Work out the finished part from the listing and answer in its coordinate system (mm). Face numbers are marked on the shaded views. A direction names the side the tool comes from. Coordinates: 2 decimals unless noted, no trailing zeros. Write each loop counter-clockwise with the first axis right and the second up, starting at its lowest first coordinate (ties: lowest second). Pieces come first, ordered by that corner, then holes. Notation, with made-up numbers: (56, 18) - (92, 18) arc R14 ccw to (92, 44) - close; hole circle Ø6 at (35.25, 58). An arc over 180 degrees is marked (long way). One line per item, written item: value.
```python
from build123d import *

# Parameters (mm, degrees)
F0_W     = 31.8
F0_H     = 15.8
F1_DEPTH = 9.6
F2_R     = 2.4
F3_DEPTH = 1.8
F4_T     = -1
F5_R     = 3.255
F5_R_2   = 2.4
F6_DEPTH = 8.6


# Not quite as in the source:
# - a pattern or mirror of a feature is missing from the dataset's text; its kind, count and spacing are read off the source's solid


with BuildPart() as f1:
    # F0 (on Top) → F1 (new body)
    with BuildSketch(Plane.XY):
        Rectangle(F0_W, F0_H)
    extrude(amount=F1_DEPTH)

    # F2 (on face) → F3 (join)
    with BuildSketch(Plane.XY.offset(9.6)):
        with Locations((-12, 4)):
            Circle(F2_R)
        with Locations((-4, 4)):
            Circle(F2_R)
        with Locations((4, 4)):
            Circle(F2_R)
        with Locations((12, 4)):
            Circle(F2_R)
    f3 = extrude(amount=F3_DEPTH)

    # F3_copies: F3 across plane
    add(f3.mirror(Plane(origin=(0, 0, 0), x_dir=(0, 0, -1), z_dir=(0, -1, 0))))

    # F4
    f4_openings = [f1.faces().sort_by_distance(p)[0] for p in [
        (0, 0, 0),
    ]]
    offset(amount=F4_T, openings=f4_openings, kind=Kind.INTERSECTION)

    # F5 (on face) → F6 (join, through all)
    with BuildSketch(Plane(origin=(0, 0, 8.6), x_dir=(1, 0, 0), z_dir=(0, 0, -1))):
        with Locations((-8, 0)):
            Circle(F5_R)
        with Locations((-8, 0)):
            Circle(F5_R_2, mode=Mode.SUBTRACT)
        Circle(F5_R)
        Circle(F5_R_2, mode=Mode.SUBTRACT)
        with Locations((8, 0)):
            Circle(F5_R)
        with Locations((8, 0)):
            Circle(F5_R_2, mode=Mode.SUBTRACT)
    extrude(amount=F6_DEPTH)


solid = f1.part
```
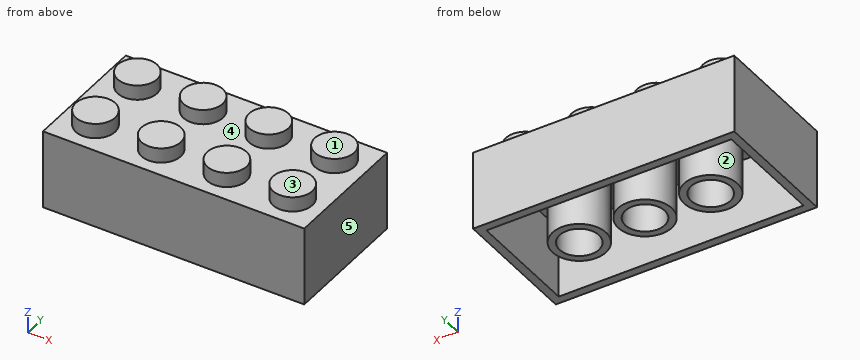
Item 1: Consider probe 1 along X at (y, z) = (4, 9.3); probe 2 along Y at (x, z) = (-8, 2.5) (3 decimals); probe 3 along Y at (x, z) = (12, 9.65). Determine where each line is inside the solid, lowest interval first.
Evaluation:
probe 1: x = -15.9 to -13.4, -10.6 to -5.4, -2.6 to 2.6, 5.4 to 10.6, 13.4 to 15.9
probe 2: y = -7.9 to -6.9, -3.255 to -2.4, 2.4 to 3.255, 6.9 to 7.9
probe 3: y = -6.4 to -5.4, -2.6 to -1.6, 1.6 to 2.6, 5.4 to 6.4
Item 2: Section A-A, the plane z = 6.5 is taken. Determine the outline of the cut face in (x, y) (3 decimals), then the cut area to 3 significant figures.
Evaluation:
outline: (-15.9, -7.9) - (15.9, -7.9) - (15.9, 7.9) - (-15.9, 7.9) - close; circle Ø6.51 at (-8, 0); circle Ø6.51 at (0, 0); circle Ø6.51 at (8, 0); hole (-14.9, -6.9) - (14.9, -6.9) - (14.9, 6.9) - (-14.9, 6.9) - close; hole circle Ø4.8 at (-8, 0); hole circle Ø4.8 at (0, 0); hole circle Ø4.8 at (8, 0)
area: 137 mm2
Item 3: Section B-B, the plane z = 9.25 is taken. Give the number of separate pieces and of enclosed holes in the cut face, then the cut area to 3 significant figures.
Evaluation:
separate pieces: 1
enclosed holes: 8
area: 453 mm2
Item 4: Section D-D, the plane x = -12 is taken. Determine the outline of the cut face in (y, z), then the cut area to 3 significant figures.
Evaluation:
outline: (-7.9, 0) - (-6.9, 0) - (-6.9, 8.6) - (-5.4, 8.6) - (-5.4, 10.4) - (-2.6, 10.4) - (-2.6, 8.6) - (2.6, 8.6) - (2.6, 10.4) - (5.4, 10.4) - (5.4, 8.6) - (6.9, 8.6) - (6.9, 0) - (7.9, 0) - (7.9, 9.6) - (6.4, 9.6) - (6.4, 11.4) - (1.6, 11.4) - (1.6, 9.6) - (-1.6, 9.6) - (-1.6, 11.4) - (-6.4, 11.4) - (-6.4, 9.6) - (-7.9, 9.6) - close
area: 40.2 mm2
Item 5: Given pin 1 (6 mm diameter, centred on x = 8, y = 0, fed in from +Z); pin 2 (2.5 mm diameter, centred on x = -1, y = -0.5, fed in from -Z); pin 3 (2.5 mm diameter, centred on x = -12, y = -4, fed in from -Z), each flat-ended and moving along its own axis, determine where each tip first touches the part or whether it passes through.
Evaluation:
pin 1: stops at z = 9.6
pin 2: stops at z = 8.6
pin 3: stops at z = 10.4
Item 6: Which of the six approach directions +Z, -Z, +X, -X, +Y, -Y give full straight-line access (tool end or side, diameter ignored) to the marked faces 1 and 2?
Evaluation:
face 1: +Z, +X, -X, +Y, -Y
face 2: -Z
Item 7: Determine the mould class of the marked faces 3, 4 and 5 for opening direction X: +X half, -X half, draft (parallel to the pull), parting line (faces both ways), or undercut.
Evaluation:
face 3: draft
face 4: undercut
face 5: +X half
